Model file for the job. Use its own axes, mm. Face numbers are marked on the shaded views. A direction names the side the tool comes from. Round coordinates to 2 decimals unless told otherwise and drop trailing zeros. Loops run counter-clockwise (first coordinate to the right, second up) from the corner with the lowest first, then second, coordinate; pieces in that order, holes last. Notation, with made-up numbers: M 89,-12 L 96,-12 A20 cw 96,6 Z; hole C 3,11.25 d4. An arc over 180 degrees is marked long. Use a Markdown table: item, result. Add a question column.
Q1. Mould opens along Y. For the marked faces 1, 2 and 3 say: +Y half, -Y half, draft (parallel to the pull), parting line (faces both ways), or undercut.
Q2. Pin check, flat tips, straight feed: pin 1 (5 mm diameter, centred on x = 70.5, y = 33, fed in from +Z); pin 2 (4 mm diameter, centred on x = 22.5, z = 13, fed in from +Y); pin 3 (1 mm diameter, centred on x = 89, y = 72.5, fed in from +Z). Stop position of each tip, or through.
Q3. Cut at B-B (x = 110). Give the cut face in (y, z).
Q4. Cut at D-D (z = 35.5). Give the cut face in (x, y).
Q5. Probe line 1 (Z direction, x = 95, y = 64); line 2 (X direction, y = 38, z = 21.5) (3 decimals); line 3 (Y direction, x = 110, z = 87.5). List the from-to ranges inside material, lowest first. Write a range as from..to.
Q6. Cut at C-C (y = 48). State how many separate pieces and enclosed holes the cut face has, plus the area to 3 significant figures.
Q7. Tool access for the marked faces 4, 5, 6 and 7: list every direction of +Z, -Z, +X, -X, +Y, -Y with a clear straight run to the whole face (end or side of a thin tool).
Q8. Cut at A-A (z = 57.5). Give the cut face in (x, y), plus the area to 3 significant figures.
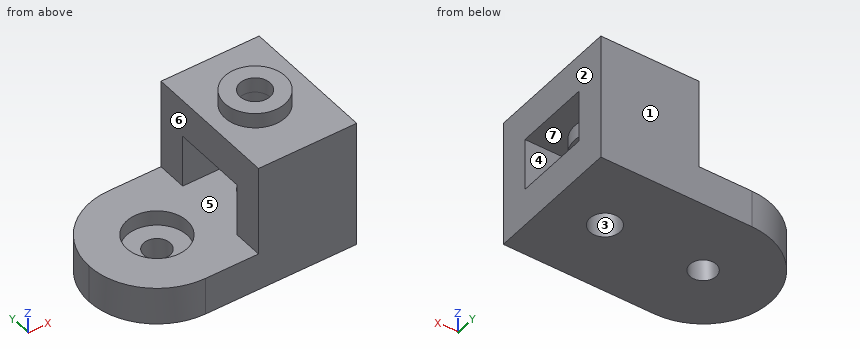
from build123d import *

# Parameters (mm, degrees)
SKETCH1_W                   = 145
SKETCH1_H                   = 90
BOSS_EXTRUDE1_DEPTH         = 85
CUT_EXTRUDE1_DEPTH          = 85
CUT_EXTRUDE3_DEPTH          = 50
M20_TAPPED_HOLE1_AT_2_COUNT = 2
M20_TAPPED_HOLE1_AT_2_PITCH = 65
M20_TAPPED_HOLE3_D          = 17.5
M20_TAPPED_HOLE3_DEPTH      = 60
M20_TAPPED_HOLE3_TIP        = 5.257530416
SKETCH12_R                  = 20
SKETCH12_R_2                = 10
CUT_EXTRUDE4_DEPTH          = 10
SKETCH13_R                  = 10
SKETCH13_R_2                = 8.75
CUT_EXTRUDE5_DEPTH          = 10
CUT_EXTRUDE6_DEPTH          = 10
SKETCH15_R                  = 20
SKETCH15_R_2                = 10
CUT_EXTRUDE7_DEPTH          = 10
SKETCH16_R                  = 10
SKETCH16_R_2                = 8.75
CUT_EXTRUDE8_DEPTH          = 10
SKETCH17_W                  = 35
SKETCH17_H                  = 50
CUT_EXTRUDE9_DEPTH          = 97
SKETCH18_R                  = 20
SKETCH18_R_2                = 10
BOSS_EXTRUDE2_DEPTH         = 10
SKETCH19_R                  = 20
SKETCH19_R_2                = 8.75
BOSS_EXTRUDE3_DEPTH         = 10
SKETCH20_R                  = 10
SKETCH20_R_2                = 8.75
CUT_EXTRUDE10_DEPTH         = 120


with BuildPart() as part:
    # Sketch1 → Boss-Extrude1 (new body)
    with BuildSketch(Plane.XY):
        with Locations((72.5, 45)):
            Rectangle(SKETCH1_W, SKETCH1_H)
    extrude(amount=BOSS_EXTRUDE1_DEPTH)

    # Sketch2 → Cut-Extrude1 (cut)
    with BuildSketch(Plane.XY.offset(85)):
        with BuildLine():
            ThreePointArc((0, 45), (13.180194847, 76.819805153), (45, 90))
            Line((45, 90), (0, 90))
            Line((0, 90), (0, 45))
        make_face()
        with BuildLine():
            ThreePointArc((45, 0), (13.180194847, 13.180194847), (0, 45))
            Line((0, 45), (0, 0))
            Line((0, 0), (45, 0))
        make_face()
    extrude(amount=-CUT_EXTRUDE1_DEPTH, mode=Mode.SUBTRACT)

    # Sketch4 → Cut-Extrude3 (cut)
    with BuildSketch(Plane.XY.offset(85)):
        with BuildLine():
            Line((80, 0), (80, 90))
            Line((80, 90), (45, 90))
            ThreePointArc((45, 90), (0, 45), (45, 0))
            Line((45, 0), (80, 0))
        make_face()
    extrude(amount=-CUT_EXTRUDE3_DEPTH, mode=Mode.SUBTRACT)

    # Sketch6 → M20 Tapped Hole1 (revolve, cut)
    with BuildSketch(Plane(origin=(45, 45, 35), x_dir=(0, -1, 0), z_dir=(1, 0, 0))):
        Polygon((0, 0), (0, 45.257530416), (8.75, 40), (8.75, 0), align=None)
    m20_tapped_hole1 = revolve(axis=Axis((45, 45, 41.35), (0, 0, -1)), mode=Mode.SUBTRACT)

    # M20 Tapped Hole1 at 2: M20 Tapped Hole1 ×2
    with Locations(*[(i * M20_TAPPED_HOLE1_AT_2_PITCH, 0, 0) for i in range(1, M20_TAPPED_HOLE1_AT_2_COUNT)]):
        add(m20_tapped_hole1, mode=Mode.SUBTRACT)

    # M20 Tapped Hole3
    with Locations(Plane(origin=(110, 45, 85), x_dir=(1, 0, 0), z_dir=(0, 0, 1))):
        with Locations((0, 0)):
            Hole(M20_TAPPED_HOLE3_D / 2, depth=M20_TAPPED_HOLE3_DEPTH)
            with Locations((0, 0, -(M20_TAPPED_HOLE3_DEPTH + M20_TAPPED_HOLE3_TIP / 2))):  # 118° drill point
                Cone(0, M20_TAPPED_HOLE3_D / 2, M20_TAPPED_HOLE3_TIP, mode=Mode.SUBTRACT)

    # Sketch12 → Cut-Extrude4 (cut)
    with BuildSketch(Plane.XY.offset(35)):
        with Locations((45, 45)):
            Circle(SKETCH12_R)
        with Locations((45, 45)):
            Circle(SKETCH12_R_2, mode=Mode.SUBTRACT)
    extrude(amount=-CUT_EXTRUDE4_DEPTH, mode=Mode.SUBTRACT)

    # Sketch13 → Cut-Extrude5 (cut)
    with BuildSketch(Plane.XY.offset(35)):
        with Locations((45, 45)):
            Circle(SKETCH13_R)
        with Locations((45, 45)):
            Circle(SKETCH13_R_2, mode=Mode.SUBTRACT)
    extrude(amount=-CUT_EXTRUDE5_DEPTH, mode=Mode.SUBTRACT)

    # Sketch14 → Cut-Extrude6 (cut)
    with BuildSketch(Plane.XY.offset(35)):
        with BuildLine():
            Line((80, 90), (80, 0))
            Line((80, 0), (45, 0))
            ThreePointArc((45, 0), (0, 45), (45, 90))
            Line((45, 90), (80, 90))
        make_face()
    extrude(amount=-CUT_EXTRUDE6_DEPTH, mode=Mode.SUBTRACT)

    # Sketch15 → Cut-Extrude7 (cut)
    with BuildSketch(Plane.XY.offset(25)):
        with Locations((45, 45)):
            Circle(SKETCH15_R)
        with Locations((45, 45)):
            Circle(SKETCH15_R_2, mode=Mode.SUBTRACT)
    extrude(amount=-CUT_EXTRUDE7_DEPTH, mode=Mode.SUBTRACT)

    # Sketch16 → Cut-Extrude8 (cut)
    with BuildSketch(Plane.XY.offset(25)):
        with Locations((45, 45)):
            Circle(SKETCH16_R)
        with Locations((45, 45)):
            Circle(SKETCH16_R_2, mode=Mode.SUBTRACT)
    extrude(amount=-CUT_EXTRUDE8_DEPTH, mode=Mode.SUBTRACT)

    # Sketch17 → Cut-Extrude9 (cut)
    with BuildSketch(Plane.ZY.offset(-80)):
        with Locations((42.5, 45)):
            Rectangle(SKETCH17_W, SKETCH17_H)
    extrude(amount=-CUT_EXTRUDE9_DEPTH, mode=Mode.SUBTRACT)

    # Sketch18 → Boss-Extrude2 (add)
    with BuildSketch(Plane.XY.offset(85)):
        with Locations((110, 45)):
            Circle(SKETCH18_R)
        with Locations((110, 45)):
            Circle(SKETCH18_R_2, mode=Mode.SUBTRACT)
    extrude(amount=BOSS_EXTRUDE2_DEPTH)

    # Sketch19 → Boss-Extrude3 (add)
    with BuildSketch(Plane(origin=(0, 0, 60), x_dir=(-1, 0, 0), z_dir=(0, 0, -1))):
        with Locations((-110, 45)):
            Circle(SKETCH19_R)
        with Locations((-110, 45)):
            Circle(SKETCH19_R_2, mode=Mode.SUBTRACT)
    extrude(amount=BOSS_EXTRUDE3_DEPTH)

    # Sketch20 → Cut-Extrude10 (cut)
    with BuildSketch(Plane.XY.offset(85)):
        with Locations((110, 45)):
            Circle(SKETCH20_R)
        with Locations((110, 45)):
            Circle(SKETCH20_R_2, mode=Mode.SUBTRACT)
    extrude(amount=-CUT_EXTRUDE10_DEPTH, mode=Mode.SUBTRACT)


solid = part.part
Checked values:
| question | item | result |
|---|---|---|
| 1 | face 1 | +Y half |
| 1 | face 2 | draft |
| 1 | face 3 | undercut |
| 2 | pin 1 | stops at z = 25 |
| 2 | pin 2 | stops at y = 85.06 |
| 2 | pin 3 | stops at z = 85 |
| 3 | outline | M 0,0 L 35,0 L 35,25 L 20,25 L 20,60 L 25,60 L 25,50 L 35,50 L 35,95 L 25,95 L 25,85 L 0,85 Z; M 55,0 L 90,0 L 90,85 L 65,85 L 65,95 L 55,95 L 55,50 L 65,50 L 65,60 L 70,60 L 70,25 L 55,25 Z |
| 4 | outline | M 80,0 L 145,0 L 145,20 L 80,20 Z; M 80,70 L 145,70 L 145,90 L 80,90 Z |
| 5 | line 1 | z = 0..25, 60..85 |
| 5 | line 2 | x = 0.548..26.265, 63.735..102.859, 117.141..145 |
| 5 | line 3 | y = 25..35, 55..65 |
| 6 | separate pieces | 5 |
| 6 | enclosed holes | 0 |
| 6 | area | 4,060 mm^2 |
| 7 | face 4 | +X, -X |
| 7 | face 5 | -X |
| 7 | face 6 | +Z, -X, +Y, -Y |
| 7 | face 7 | none |
| 8 | outline | M 80,0 L 145,0 L 145,20 L 80,20 Z; M 80,70 L 145,70 L 145,90 L 80,90 Z; C 110,45 d40; hole C 110,45 d20 |
| 8 | area | 3,540 mm^2 |
